```python
from build123d import *

# Parameters (mm, degrees)
SKETCH1_W           = 6.35
SKETCH1_H           = 25.4
BOSS_EXTRUDE1_DEPTH = 304.8
SKETCH2_R           = 5
SKETCH2_R_2         = 3.175
CUT_EXTRUDE1_DEPTH  = 306.922412549
SKETCH4_R           = 1.5
CUT_EXTRUDE2_DEPTH  = 306.922412549
SKETCH5_R           = 3.175
CUT_EXTRUDE3_DEPTH  = 306.922412549
SKETCH6_W           = 74.8
SKETCH6_H           = 25.4
CUT_EXTRUDE5_DEPTH  = 10


with BuildPart() as part:
    # Sketch1 → Boss-Extrude1 (new body)
    with BuildSketch(Plane(origin=(0, 0, 0), x_dir=(0, 0, -1), z_dir=(1, 0, 0))):
        with Locations((3.175, 12.7)):
            Rectangle(SKETCH1_W, SKETCH1_H)
    extrude(amount=BOSS_EXTRUDE1_DEPTH)

    # Sketch2 → Cut-Extrude1 (cut, through all)
    with BuildSketch(Plane.XY):
        with Locations((160.8, 12.7)):
            Circle(SKETCH2_R)
        with Locations((50.8, 12.7)):
            Circle(SKETCH2_R_2)
        with Locations((115.8, 12.7)):
            Circle(SKETCH2_R_2)
        with Locations((205.8, 12.7)):
            Circle(SKETCH2_R_2)
    extrude(amount=-CUT_EXTRUDE1_DEPTH, mode=Mode.SUBTRACT)

    # Sketch4 → Cut-Extrude2 (cut, through all)
    with BuildSketch(Plane.XY):
        with Locations((138.879689783, 20.6)):
            Circle(SKETCH4_R)
        with Locations((182.720310217, 20.6)):
            Circle(SKETCH4_R)
        with Locations((182.720310217, 4.8)):
            Circle(SKETCH4_R)
        with Locations((138.879689783, 4.8)):
            Circle(SKETCH4_R)
    extrude(amount=-CUT_EXTRUDE2_DEPTH, mode=Mode.SUBTRACT)

    # Sketch5 → Cut-Extrude3 (cut, through all)
    with BuildSketch(Plane.XY):
        with Locations((241.3, 12.7)):
            Circle(SKETCH5_R)
        with Locations((292.1, 12.7)):
            Circle(SKETCH5_R)
    extrude(amount=-CUT_EXTRUDE3_DEPTH, mode=Mode.SUBTRACT)

    # Sketch6 → Cut-Extrude5 (cut)
    with BuildSketch(Plane.XY):
        with Locations((267.4, 12.7)):
            Rectangle(SKETCH6_W, SKETCH6_H)
    extrude(amount=-CUT_EXTRUDE5_DEPTH, mode=Mode.SUBTRACT)


solid = part.part
```
The listing builds one solid part. Answer for the finished solid, in the listing's coordinates (mm). Round coordinates to 2 decimals unless told otherwise and drop trailing zeros. Loops run counter-clockwise (first coordinate to the right, second up) from the corner with the lowest first, then second, coordinate; pieces in that order, holes last.
Q1. For a pull along Y with two mould halves and no side action, classify faces 1 (the face through (113, 0, -3)), 2 (the face through (230, 13, -3)), 3 (the face through (208.73, 11.48, -3.13)) as released by +Y, released by -Y, zero draft, split by the parting line, or undercut.
Q2. Section B-B, the plane y = 12.7 is taken. Determine the outline of the cut face in (x, z) (3 decimals).
Q3. Section C-C, the plane z = -2.5 is taken. Count the separate pieces of the cut face and the enclosed holes in it, then the cut area to 3 significant figures.
Q4. Find the intervals of material crossed by line 1 (Y direction, x = 116, z = -2.25); line 2 (X direction, y = 6, z = -0.75); line 3 (Y direction, x = 160.8, z = -4.25), in increasing order.
Q5. Given pin 1 Ø4 at (x, y) = (116, 4) entering from +Z, flat-ended and moving along its own axis, determine where the tip first touches the part or whether it passes through.
Q6. Section A-A, the plane x = 115.8 is taken. Determine the outline of the cut face in (y, z) (3 decimals).
Completed:
1. face 1: released by -Y
1. face 2: zero draft
1. face 3: undercut
2. outline: (0, -6.35) - (47.625, -6.35) - (47.625, 0) - (0, 0) - close; (53.975, -6.35) - (112.625, -6.35) - (112.625, 0) - (53.975, 0) - close; (118.975, -6.35) - (155.8, -6.35) - (155.8, 0) - (118.975, 0) - close; (165.8, -6.35) - (202.625, -6.35) - (202.625, 0) - (165.8, 0) - close; (208.975, -6.35) - (230, -6.35) - (230, 0) - (208.975, 0) - close
3. separate pieces: 1
3. enclosed holes: 8
3. area: 5,640 mm2
4. line 1: y = 0 to 9.53, 15.87 to 25.4
4. line 2: x = 0 to 137.98, 139.78 to 181.82, 183.62 to 230
4. line 3: y = 0 to 7.7, 17.7 to 25.4
5. pin 1: stops at z = 0
6. outline: (0, -6.35) - (9.525, -6.35) - (9.525, 0) - (0, 0) - close; (15.875, -6.35) - (25.4, -6.35) - (25.4, 0) - (15.875, 0) - close
